Autodesk Inventor part; units mm, degrees
ref_plane "YZ Plane" through (0, 0, 0) normal (1, 0, 0) x (0, 1, 0)
ref_plane "XZ Plane" through (0, 0, 0) normal (0, 1, 0) x (-1, 0, 0)
ref_plane "XY Plane" through (0, 0, 0) normal (0, 0, 1) x (1, 0, 0)
sketch "Sketch1" plane through (0, 0, 0) normal (1, 0, 0) x (0, 1, 0)
  line L0 (52.4, 0) -> (4, 0)
  line L1 (0, -4) -> (0, -52.4)
  line L2 (4, -56.4) -> (52.4, -56.4)
  line L3 (56.4, -52.4) -> (56.4, -4)
  line L4 (51.77, -4.63) -> (4.63, -4.63) construction
  line L5 (4.63, -4.63) -> (4.63, -51.77) construction
  line L6 (4.63, -51.77) -> (51.77, -51.77) construction
  line L7 (51.77, -51.77) -> (51.77, -4.63) construction
  circle A0 centre (51.77, -4.63) radius 2.5
  circle A1 centre (51.77, -51.77) radius 2.5
  circle A2 centre (4.63, -4.63) radius 2.5
  circle A3 centre (4.63, -51.77) radius 2.5
  arc A4 (56.4, -4) -> (52.4, 0) centre (52.4, -4) ccw
  arc A5 (52.4, -56.4) -> (56.4, -52.4) centre (52.4, -52.4) ccw
  arc A6 (0, -52.4) -> (4, -56.4) centre (4, -52.4) ccw
  arc A7 (4, 0) -> (0, -4) centre (4, -4) ccw
  point P0 (0, 0)
  point P1 (56.4, 0)
  point P2 (0, 0)
  point P3 (56.4, -56.4)
  point P4 (56.4, -28.2)
  point P5 (51.77, -28.2)
  point P6 (28.2, -51.77)
  point P7 (28.2, -56.4)
  dimension "d0" = 56.4
  dimension "d1" = 47.14
  dimension "d2" = 5
  dimension "d3" = 4
  dimension "d4" = 4
  dimension "d5" = 4
  dimension "d6" = 4
extrude "Extrusion1" add sketch "Sketch1" along normal blind 112
sketch "Sketch2" plane through (0, 0, 0) normal (-1, 0, 0) x (0, 0, 1)
  circle A0 centre (-28.2, 28.2) radius 19.05
  line L0 (-52.4, 56.4) -> (-4, 56.4)
  line L1 (-56.4, 4) -> (-56.4, 52.4)
  point P0 (0, 0)
  point P1 (-28.2, 56.4)
  point P2 (-56.4, 28.2)
  dimension "d9" = 38.1
extrude "Extrusion2" add sketch "Sketch2" along normal blind 1.6
sketch "Sketch3" plane through (-1.6, 28.2, -28.2) normal (-1, 0, 0) x (0, 0, 1)
  circle A0 centre (0, 0) radius 5
  circle A1 centre (0, 0) radius 19.05 construction
  point P0 (28.2, -28.2)
  dimension "d12" = 10
extrude "Extrusion3" add sketch "Sketch3" along normal blind 24
properties part number "Nema23"
Here's how the part is built. I have some questions about the finished solid (model axes, mm). A direction names the side the tool comes from. Give positions to 0.01 mm unless a question says otherwise; leave off trailing zeros. Loops run counter-clockwise (first coordinate to the right, second up) from the corner with the lowest first, then second, coordinate; pieces in that order, holes last. Notation, with made-up numbers: M 18.25,-4 L 28.25,-4 A26 ccw 28.25,28 Z; hole C 37,67.25 d3. An arc over 180 degrees is marked long. Return JSON: item names as keys, results as strings.
Item 1: Imagine slicing it at D-D on z = -14.5. List the corners of the cut face in (x, y) for me, then the cut area to 3 significant figures.
A:
{"outline": "M -1.6,14.96 L 0,14.96 L 0,0 L 112,0 L 112,56.4 L 0,56.4 L 0,41.44 L -1.6,41.44 Z", "area": "6,360 mm^2"}
Item 2: Please list where these lines run through material, in increasing order: line 1 (Z direction, x = 53.5, y = 51.77); line 2 (Y direction, x = 27, z = -51.5); line 3 (Z direction, x = 32, y = 4).
A:
{"line 1": "z = -56.4 to -54.27, -49.27 to -7.13, -2.13 to 0", "line 2": "y = 0 to 2.14, 7.12 to 49.28, 54.26 to 56.4", "line 3": "z = -56.4 to -54.19, -49.35 to -7.05, -2.21 to 0"}
Item 3: On a 3-axis mill with a long thin cutter (end or side, diameter ignored), from which of +Z, -Z, +X, -X, +Y, -Y can I reach the whole of each face in a straight line? I mean faces 1 (the cylindrical face through (-0.789, 15.325, -42.241)), 2 (the flat face through (55, 29, 0)). Say none if no direction works.
A:
{"face 1": "-X", "face 2": "+Z, +X, -X, +Y, -Y"}
Item 4: Imagine slicing it at A-A on z = -28.2. List the corners of the cut face in (x, y) for me, then the cut area to 3 significant figures.
A:
{"outline": "M -25.6,23.2 L -1.6,23.2 L -1.6,9.15 L 0,9.15 L 0,0 L 112,0 L 112,56.4 L 0,56.4 L 0,47.25 L -1.6,47.25 L -1.6,33.2 L -25.6,33.2 Z", "area": "6,620 mm^2"}
Item 5: Imagine slicing it at B-B on x = 32.5. List the corners of the cut face in (y, z) for me.
A:
{"outline": "M 0,-52.4 A4 ccw 4,-56.4 L 52.4,-56.4 A4 ccw 56.4,-52.4 L 56.4,-4 A4 ccw 52.4,0 L 4,0 A4 ccw 0,-4 Z; hole C 4.63,-51.77 d5; hole C 4.63,-4.63 d5; hole C 51.77,-51.77 d5; hole C 51.77,-4.63 d5"}
Item 6: Thinking about a two-plate mould opening in Z: for faces 3 (the cylindrical face through (55.216, 55.197, -1.141)), 4 (the cylindrical face through (55.22, 4.09, -49.33)), 5 (the flat face through (112, 28, -28)), which applies, released by +Z, released by -Z, zero draft, split by the parting line, or undercut?
A:
{"face 3": "released by +Z", "face 4": "undercut", "face 5": "zero draft"}
Item 7: I'm going to push flat-ended pins straight in: pin 1 Ø1.5 at (x, y) = (26.5, 8.5) entering from +Z; pin 2 Ø12 at (y, z) = (19, -13) entering from -X. Where does each tip first touch, or does it pass through?
A:
{"pin 1": "stops at z = 0", "pin 2": "stops at x = -1.6"}
Item 8: Imagine slicing it at C-C on y = 28.2. List the corners of the cut face in (x, z) for me, then the cut area to 3 significant figures.
A:
{"outline": "M -25.6,-33.2 L -1.6,-33.2 L -1.6,-47.25 L 0,-47.25 L 0,-56.4 L 112,-56.4 L 112,0 L 0,0 L 0,-9.15 L -1.6,-9.15 L -1.6,-23.2 L -25.6,-23.2 Z", "area": "6,620 mm^2"}
